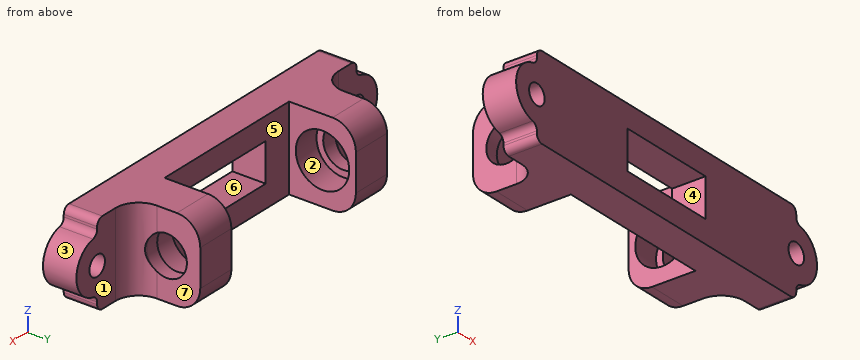
```python
from build123d import *

# Parameters (mm, degrees)
SKETCH1_R           = 1.5
BOSS_EXTRUDE1_DEPTH = 5
BOSS_EXTRUDE2_DEPTH = 10
SKETCH3_R           = 4
CUT_EXTRUDE1_DEPTH  = 4
SKETCH3_3_R         = 3
CUT_EXTRUDE2_DEPTH  = 45.102862719
FILLET6_R           = 3.5
FILLET7_R           = 3.5
FILLET8_R           = 3.5
FILLET9_R           = 3.5
FILLET10_R          = 3.5
FILLET11_R          = 3.5
FILLET12_R          = 1
FILLET13_R          = 1
FILLET14_R          = 1
FILLET15_R          = 1
FILLET16_R          = 1
FILLET17_R          = 1
FILLET18_R          = 1
FILLET19_R          = 1
SKETCH4_W           = 15
SKETCH4_H           = 5.75
CUT_EXTRUDE3_DEPTH  = 32.305949934


with BuildPart() as part:
    # Sketch1 → Boss-Extrude1 (new body)
    with BuildSketch(Plane(origin=(0, 0, 0), x_dir=(1, 0, 0), z_dir=(0, 1, 0))):
        with BuildLine():
            Line((-25, -4), (-25, -6.25))
            Line((-25, -6.25), (25, -6.25))
            Line((25, -6.25), (25, -4))
            ThreePointArc((25, -4), (29, 0), (25, 4))
            Line((25, 4), (25, 6.25))
            Line((25, 6.25), (-25, 6.25))
            Line((-25, 6.25), (-25, 4))
            ThreePointArc((-25, 4), (-29, 0), (-25, -4))
        make_face()
        with Locations(Location((25, 0, 0), (0, 0, 270))):
            Circle(SKETCH1_R, mode=Mode.SUBTRACT)
        with Locations(Location((-25, 0, 0), (0, 0, 270))):
            Circle(SKETCH1_R, mode=Mode.SUBTRACT)
    extrude(amount=BOSS_EXTRUDE1_DEPTH)

    # Sketch2 → Boss-Extrude2 (add)
    with BuildSketch(Plane(origin=(0, 5, 0), x_dir=(1, 0, 0), z_dir=(0, 1, 0))):
        Polygon((-18, 0), (-18, -6.25), (-12, -6.25), (-12, 6.25), (-18, 6.25), align=None)
    boss_extrude2 = extrude(amount=BOSS_EXTRUDE2_DEPTH)

    # Sketch3 → Cut-Extrude1 (cut)
    with BuildSketch(Plane(origin=(-12, 0, 0), x_dir=(0, 0, -1), z_dir=(1, 0, 0))):
        with Locations((0, 10)):
            Circle(SKETCH3_R)
    cut_extrude1 = extrude(amount=-CUT_EXTRUDE1_DEPTH, mode=Mode.SUBTRACT)

    # Sketch3<3> → Cut-Extrude2 (cut, through all)
    with BuildSketch(Plane(origin=(-12, 0, 0), x_dir=(0, 0, -1), z_dir=(1, 0, 0))):
        with Locations((0, 10)):
            Circle(SKETCH3_3_R)
    cut_extrude2 = extrude(amount=-CUT_EXTRUDE2_DEPTH, mode=Mode.SUBTRACT)

    # Fillet6
    # the kernel refuses this fillet: 3.5 mm, written as the material it adds along each edge
    with BuildSketch(Plane(origin=(-18, 5, -6.25), x_dir=(0, 1, 0), z_dir=(0, 0, 1))) as fillet6_piece_1_section:
        with BuildLine():
            CenterArc((FILLET6_R, FILLET6_R), FILLET6_R, 180, 90)
            Line((0, FILLET6_R), (0, 0))
            Line((0, 0), (FILLET6_R, 0))
        make_face()
    fillet6_piece_1 = extrude(amount=12.5, mode=Mode.PRIVATE)
    fillet6_piece_1 = fillet6_piece_1 - Plane(origin=(-18.808785758, 10, 0), x_dir=(0, 0, -1), z_dir=(1, 0, 0)) * Cylinder(3, 39, mode=Mode.PRIVATE)
    add(fillet6_piece_1)

    # Fillet7
    fillet7_edges = [part.edges().sort_by_distance(p)[0] for p in [
        (-15, 15, -6.25),
    ]]
    fillet(fillet7_edges, radius=FILLET7_R)

    # Fillet8
    fillet8_edges = [part.edges().sort_by_distance(p)[0] for p in [
        (-15, 15, 6.25),
    ]]
    fillet(fillet8_edges, radius=FILLET8_R)

    # Mirror4: Boss-Extrude2, Cut-Extrude1, Cut-Extrude2 across plane
    add(boss_extrude2.mirror(Plane(origin=(0, 0, 0), x_dir=(0, 0, 1), z_dir=(1, 0, 0))))
    add(cut_extrude1.mirror(Plane(origin=(0, 0, 0), x_dir=(0, 0, 1), z_dir=(1, 0, 0))), mode=Mode.SUBTRACT)
    add(cut_extrude2.mirror(Plane(origin=(0, 0, 0), x_dir=(0, 0, 1), z_dir=(1, 0, 0))), mode=Mode.SUBTRACT)

    # Fillet9
    fillet9_edges = [part.edges().sort_by_distance(p)[0] for p in [
        (15, 15, -6.25),
    ]]
    fillet(fillet9_edges, radius=FILLET9_R)

    # Fillet10
    fillet10_edges = [part.edges().sort_by_distance(p)[0] for p in [
        (15, 15, 6.25),
    ]]
    fillet(fillet10_edges, radius=FILLET10_R)

    # Fillet11
    # the kernel refuses this fillet: 3.5 mm, written as the material it adds along each edge
    with BuildSketch(Plane(origin=(18, 5, -6.25), x_dir=(0, 1, 0), z_dir=(0, 0, 1))) as fillet11_piece_1_section:
        with BuildLine():
            CenterArc((FILLET11_R, -FILLET11_R), FILLET11_R, 90, 90)
            Line((0, -FILLET11_R), (0, 0))
            Line((0, 0), (FILLET11_R, 0))
        make_face()
    fillet11_piece_1 = extrude(amount=12.5, mode=Mode.PRIVATE)
    fillet11_piece_1 = fillet11_piece_1 - Plane(origin=(18.808785758, 10, 0), x_dir=(0, 0, -1), z_dir=(-1, 0, 0)) * Cylinder(3, 39, mode=Mode.PRIVATE)
    add(fillet11_piece_1)

    # Fillet12
    fillet12_edges = [part.edges().sort_by_distance(p)[0] for p in [
        (25, 2.5, -6.25),
    ]]
    fillet(fillet12_edges, radius=FILLET12_R)

    # Fillet13
    fillet13_edges = [part.edges().sort_by_distance(p)[0] for p in [
        (25, 2.5, 6.25),
    ]]
    fillet(fillet13_edges, radius=FILLET13_R)

    # Fillet14
    fillet14_edges = [part.edges().sort_by_distance(p)[0] for p in [
        (-25, 2.5, 6.25),
    ]]
    fillet(fillet14_edges, radius=FILLET14_R)

    # Fillet15
    fillet15_edges = [part.edges().sort_by_distance(p)[0] for p in [
        (-25, 2.5, -6.25),
    ]]
    fillet(fillet15_edges, radius=FILLET15_R)

    # Fillet16
    fillet16_edges = [part.edges().sort_by_distance(p)[0] for p in [
        (-25, 2.5, -4),
    ]]
    fillet(fillet16_edges, radius=FILLET16_R)

    # Fillet17
    fillet17_edges = [part.edges().sort_by_distance(p)[0] for p in [
        (-25, 2.5, 4),
    ]]
    fillet(fillet17_edges, radius=FILLET17_R)

    # Fillet18
    fillet18_edges = [part.edges().sort_by_distance(p)[0] for p in [
        (25, 2.5, 4),
    ]]
    fillet(fillet18_edges, radius=FILLET18_R)

    # Fillet19
    fillet19_edges = [part.edges().sort_by_distance(p)[0] for p in [
        (25, 2.5, -4),
    ]]
    fillet(fillet19_edges, radius=FILLET19_R)

    # Sketch4 → Cut-Extrude3 (cut, through all)
    with BuildSketch(Plane(origin=(0, 5, 0), x_dir=(1, 0, 0), z_dir=(0, 1, 0))):
        Rectangle(SKETCH4_W, SKETCH4_H)
    extrude(amount=-CUT_EXTRUDE3_DEPTH, mode=Mode.SUBTRACT)


solid = part.part
```
The listing builds one solid part. Answer for the finished solid, in the listing's coordinates (mm). Face numbers are marked on the shaded views. A direction names the side the tool comes from. Give positions to 0.01 mm unless a question says otherwise; leave off trailing zeros. Order: outer loops, then holes, each group sorted by start corner. A loop starts at its lowest first (then second) coordinate and runs counter-clockwise, first axis right, second up. Notation, with made-up numbers: (81, 4) -> (107, 4) arc R12 ccw to (107, 22) -> close; hole circle Ø3 at (22, 47.25). An arc over 180 degrees is marked (long way). Answer as CSV lines item,"result". Start each with the question number.
Q1. Find the intervals of material crossed by L1, parallel to Y at x = -17.4, z = 0; L2, parallel to Z at x = -6, y = 4.75 (3 decimals); L3, parallel to X at y = 13.75, z = -0.25, in increasing order.
Q2. Which of the six approach directions +Z, -Z, +X, -X, +Y, -Y give full straight-line access (tool end or side, diameter ignored) to the marked faces 5, 6 and 7?
Q3. Given pin 1 (3 mm diameter, centred on y = 13, z = 0.5, fed in from +X); pin 2 (7 mm diameter, centred on y = 10, z = 0, fed in from +X); pin 3 (2 mm diameter, centred on x = 24.5, z = -1, fed in from +Y); pin 4 (1.5 mm diameter, centred on y = 10.5, z = 0.5, fed in from +X), each flat-ended and moving along its own axis, determine where each tip first touches the part or whether it passes through.
Q4. A cutting plane is placed at D-D (y = 10). Determine the outline of the cut face in (x, z).
Q5. Determine the mould class of the marked faces 1, 2, 3 and 4 for opening direction Z: pulls with the +Z half, pulls with the -Z half, needs draft (parallel to the pull), parting line crosses it, or undercut.
Q6. A cutting plane is placed at A-A (x = -2.5). Determine the outline of the cut face in (y, z) (3 decimals).
Q7. A cutting plane is placed at C-C (x = -13). Determine the outline of the cut face in (y, z), then the cut area to 3 significant figures.
Q8. A cutting plane is placed at B-B (y = 4.25). Determine the outline of the cut face in (x, z) (3 decimals), then the cut area to 3 significant figures.
Results found:
1,L1,"0 to 7, 13 to 15"
1,L2,"-6.25 to -2.875, 2.875 to 6.25"
1,L3,"-18 to -16, 16 to 18"
2,face 5,"+Z, -Z, +Y"
2,face 6,"+Y, -Y"
2,face 7,"+Z, -Z, +X, +Y"
3,pin 1,"x = 18"
3,pin 2,"x = 18.63"
3,pin 3,"y = 5"
3,pin 4,"through"
4,outline,"(-18, -6.25) -> (-12, -6.25) -> (-12, -4) -> (-16, -4) -> (-16, -3) -> (-18, -3) -> close; (-18, 3) -> (-16, 3) -> (-16, 4) -> (-12, 4) -> (-12, 6.25) -> (-18, 6.25) -> close; (12, -6.25) -> (18, -6.25) -> (18, -3) -> (16, -3) -> (16, -4) -> (12, -4) -> close; (12, 4) -> (16, 4) -> (16, 3) -> (18, 3) -> (18, 6.25) -> (12, 6.25) -> close"
5,face 1,"needs draft"
5,face 2,"undercut"
5,face 3,"parting line crosses it"
5,face 4,"undercut"
6,outline,"(0, -6.25) -> (5, -6.25) -> (5, -2.875) -> (0, -2.875) -> close; (0, 2.875) -> (5, 2.875) -> (5, 6.25) -> (0, 6.25) -> close"
7,outline,"(0, -6.25) -> (11.5, -6.25) arc R3.5 ccw to (15, -2.75) -> (15, 2.75) arc R3.5 ccw to (11.5, 6.25) -> (0, 6.25) -> close; hole circle Ø8 at (10, 0)"
7,area,"132 mm2"
8,outline,"(-25.8, -3.919) arc R1 cw to (-25, -4.899) -> (-25, -5.25) arc R1 ccw to (-24, -6.25) -> (24, -6.25) arc R1 ccw to (25, -5.25) -> (25, -4.899) arc R1 cw to (25.8, -3.919) arc R4 ccw to (25.8, 3.919) arc R1 cw to (25, 4.899) -> (25, 5.25) arc R1 ccw to (24, 6.25) -> (-24, 6.25) arc R1 ccw to (-25, 5.25) -> (-25, 4.899) arc R1 cw to (-25.8, 3.919) arc R4 ccw to start; hole circle Ø3 at (-25, 0); hole (-7.5, -2.875) -> (7.5, -2.875) -> (7.5, 2.875) -> (-7.5, 2.875) -> close; hole circle Ø3 at (25, 0)"
8,area,"575 mm2"
